Here's how the part is built. I have some questions about the finished solid (model axes, mm). A direction names the side the tool comes from. Round coordinates to 2 decimals unless told otherwise and drop trailing zeros. Order: outer loops, then holes, each group sorted by start corner. A loop starts at its lowest first (then second) coordinate and runs counter-clockwise, first axis right, second up. Notation, with made-up numbers: (-20, 6) -> (33, 6) arc R17 ccw to (33, 18) -> close; hole circle Ø10 at (-15, 9). An arc over 180 degrees is marked (long way). One line per item, written item: value.
```python
from build123d import *

# Parameters (mm, degrees)
SKETCH_2_R               = 0.5
SKETCH_2_W               = 1
SKETCH_2_H               = 4
CUT_EXTRUDE_1_DEPTH      = 7.5
PATTERN_CIRCULAR_1_COUNT = 20
SKETCH_3_R               = 2.5
CUT_EXTRUDE_2_DEPTH      = 20.595917942


with BuildPart() as part:
    # 草图1 → 旋转3 (revolve)
    with BuildSketch(Plane.XY, mode=Mode.PRIVATE) as revolve_3_sk:
        Polygon((-8, 0), (0, 0), (0, -16), (-8, -16), (-8, -8.5), (-6, -8.5), (-6, -1), (-8, -1), align=None)
    revolve(revolve_3_sk.sketch.rotate(Axis((0, 0, 0), (0, 1, 0)), 270), axis=Axis((0, 0, 0), (0, 1, 0)))

    # 草图2 → 切除-拉伸1 (cut)
    with BuildSketch(Plane.XZ.offset(1)):
        with Locations((0, 5)):
            Circle(SKETCH_2_R)
        with Locations((0, 7)):
            Rectangle(SKETCH_2_W, SKETCH_2_H)
    cut_extrude_1 = extrude(amount=CUT_EXTRUDE_1_DEPTH, mode=Mode.SUBTRACT)

    # 阵列(圆周)1: 切除-拉伸1 ×20 about axis
    pattern_circular_1_axis = Axis((0, 0, 0), (0, 1, 0))
    for i in range(1, PATTERN_CIRCULAR_1_COUNT):
        add(cut_extrude_1.rotate(pattern_circular_1_axis, i * 360 / PATTERN_CIRCULAR_1_COUNT), mode=Mode.SUBTRACT)

    # 草图3 → 切除-拉伸2 (cut, through all)
    with BuildSketch(Plane(origin=(0, 0, 0), x_dir=(1, 0, 0), z_dir=(0, 1, 0))):
        with Locations(Location((0, 0, 0), (0, 0, 270))):
            Circle(SKETCH_3_R)
    extrude(amount=-CUT_EXTRUDE_2_DEPTH, mode=Mode.SUBTRACT)


solid = part.part
```
Q1. I want a section at D-D on x = -6.5. Write out the boundary of the cut face in (y, z).
Answers:
outline: (-16, -4.66) -> (-8.5, -4.66) -> (-8.5, 4.66) -> (-16, 4.66) -> close; (-1, -4.66) -> (0, -4.66) -> (0, 4.66) -> (-1, 4.66) -> close
Q2. Which directions (+Z, -Z, +X, -X, +Y, -Y) give clear straight access to the entire face, cutting with the end or side of a thin tool? Please do faces 1 (the face through (4.5, -4.7, 0)), 2 (the face through (0, -4.7, 4.5)), 3 (the face through (0, -1, 5)).
Answers:
face 1: +X
face 2: +Z
face 3: none
Q3. I want a section at C-C on y = -12.5. Write out the boundary of the cut face in (x, z).
Answers:
outline: circle Ø16 at (0, 0); hole circle Ø5 at (0, 0)
Q4. I want a section at B-B on z = 0. Write out the boundary of the cut face in (x, y), then the cut area to 4 significant figures.
Answers:
outline: (-8, -16) -> (-2.5, -16) -> (-2.5, 0) -> (-8, 0) -> (-8, -1) -> (-4.5, -1) -> (-4.5, -8.5) -> (-8, -8.5) -> close; (2.5, -16) -> (8, -16) -> (8, -8.5) -> (4.5, -8.5) -> (4.5, -1) -> (8, -1) -> (8, 0) -> (2.5, 0) -> close
area: 123.5 mm2
Q5. If we mould it in two halves opening along Z, with no side actions, what happens to faces 4 (the face through (-5.925, -4.698, -0.945)), 5 (the face through (-1.22, -4.7, 5.37)), 6 (the face through (-0.945, -4.698, 5.925))? For each: pulls with the +Z half, pulls with the -Z half, needs draft (parallel to the pull), parting line crosses it, or undercut.
Answers:
face 4: pulls with the -Z half
face 5: undercut
face 6: pulls with the +Z half
Q6. I want a section at A-A on x = 0. Write out the boundary of the cut face in (y, z).
Answers:
outline: (-16, -8) -> (-8.5, -8) -> (-8.5, -4.5) -> (-1, -4.5) -> (-1, -8) -> (0, -8) -> (0, -2.5) -> (-16, -2.5) -> close; (-16, 2.5) -> (0, 2.5) -> (0, 8) -> (-1, 8) -> (-1, 4.5) -> (-8.5, 4.5) -> (-8.5, 8) -> (-16, 8) -> close
Q7. I need wall thicknesses on line 1 along Y through (x, z) = (0.25, 5.5); line 2 along X through (y, z) = (-6.5, 0); line 3 along X through (y, z) = (-11, 0). Which ranges of each line are inside material? Lowest first, please.
Answers:
line 1: -16 to -8.5, -1 to 0
line 2: -4.5 to -2.5, 2.5 to 4.5
line 3: -8 to -2.5, 2.5 to 8
Q8. For P1, Ø0.5, axis at y = -6.5, z = 5.5, coming from the -X side; P2, Ø1, axis at y = -7.5, z = -2, coming from the +X side; P3, Ø6, axis at x = -4, z = 2.5, coming from the +Y side; P4, Ø2, axis at y = -12, z = 4, coming from the -X side, each with a flat end and sliding along its axis, tell me the tip position at first contact or that it passes through.
Answers:
P1: x = -2.9
P2: x = 5.53
P3: y = 0
P4: x = -7.42
